Here's how the part is built. I have some questions about the finished solid (model axes, mm). Face numbers are marked on the shaded views. A direction names the side the tool comes from. Round coordinates to 2 decimals unless told otherwise and drop trailing zeros. Order: outer loops, then holes, each group sorted by start corner. A loop starts at its lowest first (then second) coordinate and runs counter-clockwise, first axis right, second up.
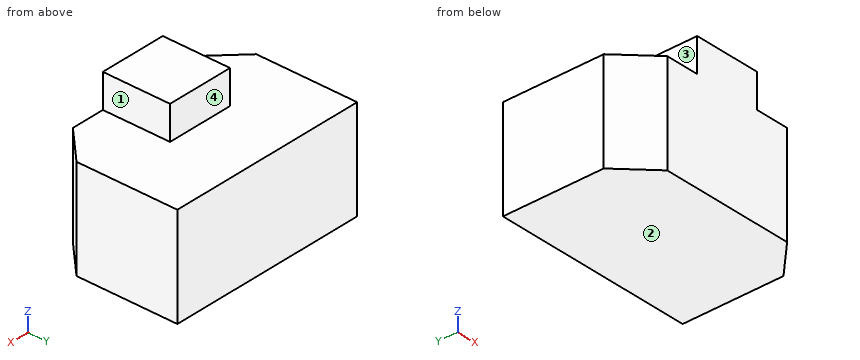
```python
from build123d import *

# Parameters (mm, degrees)
F1_DEPTH = 76.2
F3_W     = 50.8
F3_H     = 50.8
F4_DEPTH = 25.4


with BuildPart() as f1:
    # F0 (on Top) → F1 (new body)
    with BuildSketch(Plane.XY):
        Polygon((76.2, 50.8), (-76.2, 50.8), (-76.2, -25.4), (-50.8, -50.8), (50.8, -50.8), (76.2, -25.4), align=None)
    extrude(amount=F1_DEPTH)

    # F3 (on offset) → F4 (join)
    with BuildSketch(Plane.XY.offset(76.2)):
        with Locations((0, -25.4)):
            Rectangle(F3_W, F3_H)
    extrude(amount=F4_DEPTH)


solid = f1.part
```
1. On a 3-axis mill with a long thin cutter (end or side, diameter ignored), from which of +Z, -Z, +X, -X, +Y, -Y can I reach the whole of each face in a straight line? I mean the marked faces 1, 2, 3 and 4. Say none if no direction works.
Evaluation:
face 1: +Z, +X, +Y, -Y
face 2: -Z, +X, -X, +Y, -Y
face 3: +Z, -X, +Y, -Y
face 4: +Z, +X, -X, +Y
2. If we section it at D-D, the plane y = -42: Write out the boundary of the cut face in (x, z), and give its area (3 significant figures).
Evaluation:
outline: (-59.6, 0) - (59.6, 0) - (59.6, 76.2) - (25.4, 76.2) - (25.4, 101.6) - (-25.4, 101.6) - (-25.4, 76.2) - (-59.6, 76.2) - close
area: 10,400 mm2
3. If we section it at A-A, the plane y = -31: Write out the boundary of the cut face in (x, z).
Evaluation:
outline: (-70.6, 0) - (70.6, 0) - (70.6, 76.2) - (25.4, 76.2) - (25.4, 101.6) - (-25.4, 101.6) - (-25.4, 76.2) - (-70.6, 76.2) - close
4. If we section it at B-B, the plane x = 17: Write out the boundary of the cut face in (y, z).
Evaluation:
outline: (-50.8, 0) - (50.8, 0) - (50.8, 76.2) - (0, 76.2) - (0, 101.6) - (-50.8, 101.6) - close
5. I'm going to push a flat-ended pin straight in: P1, Ø20.5, axis at y = -31, z = 90, coming from the +X side. Where does the tip first touch, or does it pass through?
Evaluation:
P1: stops at x = 25.4
6. I need wall thicknesses on probe 1 along Z at (x, y) = (-8, 25.5); probe 2 along Y at (x, z) = (17.5, 88.5); probe 3 along X at (y, z) = (-23.5, 84.5). Which ranges of each line are inside material? Lowest first, please.
Evaluation:
probe 1: z = 0 to 76.2
probe 2: y = -50.8 to 0
probe 3: x = -25.4 to 25.4
7. If we section it at C-C, the plane z = 26.5: Write out the boundary of the cut face in (x, y).
Evaluation:
outline: (-76.2, -25.4) - (-50.8, -50.8) - (50.8, -50.8) - (76.2, -25.4) - (76.2, 50.8) - (-76.2, 50.8) - close
